from build123d import *

# Parameters (mm, degrees)
SKETCH1_R           = 28.5
SKETCH1_R_2         = 21
BOSS_EXTRUDE1_DEPTH = 61.675
SKETCH2_R           = 2.25
CUT_EXTRUDE1_DEPTH  = 74.677035941
CIRPATTERN1_COUNT   = 4
SKETCH3_R           = 2.25
CUT_EXTRUDE2_DEPTH  = 6.5


with BuildPart() as part:
    # Sketch1 → Boss-Extrude1 (new, symmetric)
    with BuildSketch(Plane(origin=(0, 0, 0), x_dir=(1, 0, 0), z_dir=(0, 1, 0))):
        with Locations(Location((0, 0, 0), (0, 0, 270))):
            Circle(SKETCH1_R)
        with Locations(Location((0, 0, 0), (0, 0, 270))):
            Circle(SKETCH1_R_2, mode=Mode.SUBTRACT)
    extrude(amount=BOSS_EXTRUDE1_DEPTH, both=True)

    # Sketch2 → Cut-Extrude1 (cut, through all)
    with BuildSketch(Plane.XY):
        with Locations(Location((0, 56.675, 0), (0, 0, 90))):
            Circle(SKETCH2_R)
    cut_extrude1 = extrude(amount=-CUT_EXTRUDE1_DEPTH, mode=Mode.SUBTRACT)

    # CirPattern1: Cut-Extrude1 ×4 about axis
    cirpattern1_axis = Axis((0, 61.675, 0), (0, -1, 0))
    for i in range(1, CIRPATTERN1_COUNT):
        add(cut_extrude1.rotate(cirpattern1_axis, i * 360 / CIRPATTERN1_COUNT), mode=Mode.SUBTRACT)

    # Sketch3 → Cut-Extrude2 (cut)
    with BuildSketch(Plane.XZ.offset(61.675)):
        with Locations(Location((0, 24.75, 0), (0, 0, 270))):
            Circle(SKETCH3_R)
        with Locations(Location((24.75, 0, 0), (0, 0, 270))):
            Circle(SKETCH3_R)
        with Locations(Location((0, -24.75, 0), (0, 0, 270))):
            Circle(SKETCH3_R)
        with Locations(Location((-24.75, 0, 0), (0, 0, 270))):
            Circle(SKETCH3_R)
    extrude(amount=-CUT_EXTRUDE2_DEPTH, mode=Mode.SUBTRACT)


solid = part.part
For this review, take the finished solid that the model builds, in its own axes (mm). A direction names the side the tool comes from. Round coordinates to 2 decimals unless told otherwise and drop trailing zeros. Write each loop counter-clockwise with the first axis right and the second up, starting at its lowest first coordinate (ties: lowest second). Pieces come first, ordered by that corner, then holes. Notation, with made-up numbers: (10.5, -7.5) -> (50.5, -7.5) arc R18 ccw to (50.5, 7.5) -> close; hole circle Ø9 at (71, -29). An arc over 180 degrees is marked (long way). Use CSV: the item, a comma, the result in double quotes.
(1) Clearance check with flat-ended pins moving along their axes: P1, Ø12, axis at x = 21.5, y = -24.5, coming from the -Z side; P2, Ø1.3, axis at x = 24, z = 0, coming from the -Y side (3 decimals); P3, Ø8, axis at x = -21, y = -36.5, coming from the +Z side. State where each tip first meets the part, or that it passes through.
Computed values:
P1,"z = -23.92"
P2,"y = -55.175"
P3,"z = 22.87"
(2) Consider section D-D, the plane y = 22. Give the boundary of the cut face in (x, z).
Computed values:
outline,"circle Ø57 at (0, 0); hole circle Ø42 at (0, 0)"
(3) Consider section B-B, the plane z = 0. Give the boundary of the cut face in (x, y) (3 decimals).
Computed values:
outline,"(-28.5, -61.675) -> (-27, -61.675) -> (-27, -55.175) -> (-22.5, -55.175) -> (-22.5, -61.675) -> (-21, -61.675) -> (-21, 54.425) -> (-28.5, 54.425) -> close; (-28.5, 58.925) -> (-21, 58.925) -> (-21, 61.675) -> (-28.5, 61.675) -> close; (21, -61.675) -> (22.5, -61.675) -> (22.5, -55.175) -> (27, -55.175) -> (27, -61.675) -> (28.5, -61.675) -> (28.5, 54.425) -> (21, 54.425) -> close; (21, 58.925) -> (28.5, 58.925) -> (28.5, 61.675) -> (21, 61.675) -> close"
(4) Draft analysis for pull direction Y (two halves, no side actions). For faces 1 (the face through (-0.862, 58.753, 24.636)), 2 (the face through (0.676, -58.47, 22.604)), 3 (the face through (0, -55.175, -25)), state which applies: +Y half, -Y half, draft (parallel to the pull), parting line (faces both ways), or undercut.
Computed values:
face 1,"undercut"
face 2,"draft"
face 3,"-Y half"
(5) For faces 4 (the face through (0.676, -58.47, -26.896)), 5 (the face through (-17, 61.675, -13)), list the 3-axis set-ups (+Z, -Z, +X, -X, +Y, -Y) from which the entire face can be reached by the end or side of a thin tool; tool diameter is ignored.
Computed values:
face 4,"-Y"
face 5,"+Z, -Z, +X, -X, +Y"
(6) To check wall thickness, follow L1, parallel to X at y = -60.5, z = 0; L2, parallel to X at y = 3, z = 1; L3, parallel to Z at x = 0, y = -2.5. State the ranges of each line that lie inside material, in increasing order. Write a range as [from, to].
Computed values:
L1,"[-28.5, -27], [-22.5, -21], [21, 22.5], [27, 28.5]"
L2,"[-28.48, -20.98], [20.98, 28.48]"
L3,"[-28.5, -21], [21, 28.5]"
(7) Consider section A-A, the plane x = 0. Give the boundary of the cut face in (y, z) (3 decimals).
Computed values:
outline,"(-61.675, -28.5) -> (54.425, -28.5) -> (54.425, -21) -> (-61.675, -21) -> (-61.675, -22.5) -> (-55.175, -22.5) -> (-55.175, -27) -> (-61.675, -27) -> close; (-61.675, 21) -> (54.425, 21) -> (54.425, 28.5) -> (-61.675, 28.5) -> (-61.675, 27) -> (-55.175, 27) -> (-55.175, 22.5) -> (-61.675, 22.5) -> close; (58.925, -28.5) -> (61.675, -28.5) -> (61.675, -21) -> (58.925, -21) -> close; (58.925, 21) -> (61.675, 21) -> (61.675, 28.5) -> (58.925, 28.5) -> close"
(8) Consider section C-C, the plane z = 10.5. Give the boundary of the cut face in (x, y) (3 decimals), plus the area to 3 significant figures.
Computed values:
outline,"(-26.495, -61.675) -> (-18.187, -61.675) -> (-18.187, 61.675) -> (-26.495, 61.675) -> close; (18.187, -61.675) -> (26.495, -61.675) -> (26.495, 61.675) -> (18.187, 61.675) -> close"
area,"2,050 mm²"
